from build123d import *

# Parameters (mm, degrees)
BASE_FLANGE1_DEPTH      = 1.51892
HEM1_START              = -12.7
HEM1_DEPTH              = 25.4
HEM1_2_DEPTH            = 5.08
HEM1_START_2            = 7.62
HEM1_3_DEPTH            = 5.08
CUT_EXTRUDE1_DEPTH      = 42.243563617
CUT_EXTRUDE1_DEPTH_BACK = 42.243563617


# Read off the part's stored shape, not the designer's step: Hem1
# Sheet-metal steps are written as plain solids
with BuildPart() as part:
    # Sketch1 → Base-Flange1 (new body)
    with BuildSketch(Plane.XY):
        with BuildLine():
            Line((38.1, -7.62), (38.1, -12.7))
            Line((38.1, -12.7), (-31.75, -12.7))
            ThreePointArc((-31.75, -12.7), (-36.240128061, -10.840128061), (-38.1, -6.35))
            Line((-38.1, -6.35), (-38.1, 6.35))
            ThreePointArc((-38.1, 6.35), (-36.240128061, 10.840128061), (-31.75, 12.7))
            Line((-31.75, 12.7), (38.1, 12.7))
            Line((38.1, 12.7), (38.1, 7.62))
            Line((38.1, 7.62), (25.4, 7.62))
            Line((25.4, 7.62), (25.4, -7.62))
            Line((25.4, -7.62), (38.1, -7.62))
        make_face()
    extrude(amount=-BASE_FLANGE1_DEPTH)

    # Hem1 outline → Hem1 (cut)
    with BuildSketch(Plane(origin=(0, 0, 0), x_dir=(1, 0, 0), z_dir=(0, 1, 0)).offset(HEM1_START)):
        with BuildLine():
            Line((38.1, 1.51892), (36.863284068, 1.51892))
            ThreePointArc((36.863284068, 1.51892), (35.294159576, 0.396474191), (33.40608, 0))
            Line((33.40608, 0), (38.1, 0))
            Line((38.1, 0), (38.1, 1.51892))
        make_face()
    extrude(amount=HEM1_DEPTH, mode=Mode.SUBTRACT)

    # Hem1 2 outline → Hem1 2 (add)
    with BuildSketch(Plane(origin=(0, 0, 0), x_dir=(1, 0, 0), z_dir=(0, 1, 0)).offset(HEM1_START)):
        with BuildLine():
            Line((29.341026037, 2.34696), (30.656449343, 3.10642))
            ThreePointArc((30.656449343, 3.10642), (34.99358, 7.443550657), (33.40608, 1.51892))
            Line((33.40608, 1.51892), (36.863284068, 1.51892))
            ThreePointArc((36.863284068, 1.51892), (33.919678028, 9.359657029), (29.341026037, 2.34696))
        make_face()
    extrude(amount=HEM1_2_DEPTH)

    # Hem1 3 outline → Hem1 3 (add)
    with BuildSketch(Plane(origin=(0, 0, 0), x_dir=(1, 0, 0), z_dir=(0, 1, 0)).offset(HEM1_START_2)):
        with BuildLine():
            Line((29.341026037, 2.34696), (30.656449343, 3.10642))
            ThreePointArc((30.656449343, 3.10642), (34.99358, 7.443550657), (33.40608, 1.51892))
            Line((33.40608, 1.51892), (36.863284068, 1.51892))
            ThreePointArc((36.863284068, 1.51892), (33.919678028, 9.359657029), (29.341026037, 2.34696))
        make_face()
    extrude(amount=HEM1_3_DEPTH)

    # Sketch8 → Cut-Extrude1 (cut, two sides: drawn at the far end of the back side and taken through both)
    with BuildSketch(Plane.XY.offset(-CUT_EXTRUDE1_DEPTH_BACK)):
        with BuildLine():
            Line((-33.02, 2.54), (-2.54, 2.54))
            ThreePointArc((-2.54, 2.54), (0, 0), (-2.54, -2.54))
            Line((-2.54, -2.54), (-33.02, -2.54))
            ThreePointArc((-33.02, -2.54), (-35.56, 0), (-33.02, 2.54))
        make_face()
    extrude(amount=CUT_EXTRUDE1_DEPTH + CUT_EXTRUDE1_DEPTH_BACK, mode=Mode.SUBTRACT)


solid = part.part
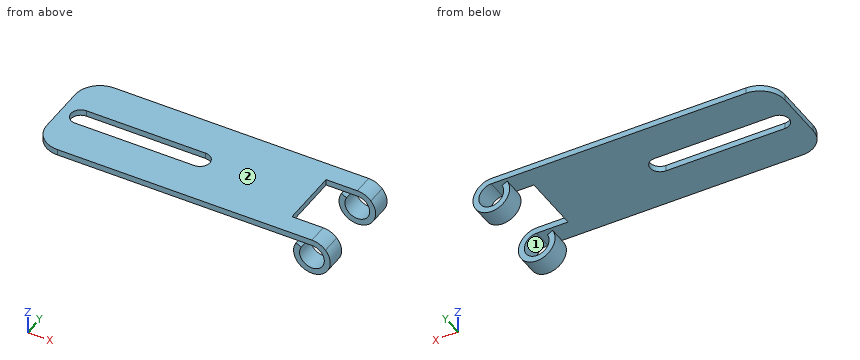
Build history of the part. All positions in model axes, mm. Face numbers are marked on the shaded views. Coordinates: 2 decimals unless noted, no trailing zeros. Order: outer loops, then holes, each group sorted by start corner. A loop starts at its lowest first (then second) coordinate and runs counter-clockwise, first axis right, second up. Notation, with made-up numbers: (65, 55) - (118, 55) arc R24 ccw to (118, 72) - close; hole circle Ø8 at (-2, 86.5). An arc over 180 degrees is marked (long way). Write item = value, one per line. Start each with the question number.
1) Saw through at C-C on y = 9.5. Write the cut outline in (x, z) (3 decimals).
2) Flat gauge pins, fed straight in: pin 1 Ø1.5 at (y, z) = (9, -4.5) entering from -X; pin 2 Ø1.2 at (y, z) = (3.5, -0.5) entering from +X; pin 3 Ø2 at (x, y) = (28.5, 10) entering from -Z; pin 4 Ø3 at (x, z) = (-3.5, -3.5) entering from +Y. Where does each tip first touch, or does it go through?
3) Saw through at B-B on z = -5.5. Write the cut outline in (x, y).
4) Wall check: line 1 along Z through (x, y) = (30.5, -9.75); line 2 along X through (y, z) = (-4.75, -1.25); line 3 along Z through (x, y) = (-6.5, -10). Give the ranges that are in metal, low to high. Write a range as from..to.
5) Saw through at D-D on x = 15.5. Write the cut outline in (y, z).
6) Saw through at A-A on y = 0. Write the cut outline in (x, z), then the cut area to 3 significant figures.
7) Two-plate mould, pull along Z, no slides. Class the marked faces 1 and 2: pulls with the +Z half, pulls with the -Z half, needs draft (parallel to the pull), parting line crosses it, or undercut.
From the geometry:
q1.outline = (-37.264, -1.519) - (33.406, -1.519) arc R3.175 cw (long way) to (30.656, -3.106) - (29.341, -2.347) arc R4.694 ccw (long way) to (33.406, 0) - (-37.264, 0) - close
q2.pin_1 = 28.71
q2.pin_2 = 25.4
q2.pin_3 = -7.3
q2.pin_4 = through
q3.outline = (28.78, -12.7) - (30.34, -12.7) - (30.34, -7.62) - (28.78, -7.62) - close; (28.78, 7.62) - (30.34, 7.62) - (30.34, 12.7) - (28.78, 12.7) - close; (36.48, -12.7) - (38.03, -12.7) - (38.03, -7.62) - (36.48, -7.62) - close; (36.48, 7.62) - (38.03, 7.62) - (38.03, 12.7) - (36.48, 12.7) - close
q4.line_1 = -8.38..-5.97, -3.42..-3.02, -1.52..0
q4.line_2 = -38.1..25.4
q4.line_3 = -1.52..0
q5.outline = (-12.7, -1.52) - (12.7, -1.52) - (12.7, 0) - (-12.7, 0) - close
q6.outline = (-38.1, -1.52) - (-35.56, -1.52) - (-35.56, 0) - (-38.1, 0) - close; (0, -1.52) - (25.4, -1.52) - (25.4, 0) - (0, 0) - close
q6.area = 42.4 mm^2
q7.face_1 = undercut
q7.face_2 = pulls with the +Z half
